from build123d import *

# Parameters (mm, degrees)
SKETCH1_W                          = 20
SKETCH1_H                          = 25
BOSS_EXTRUDE1_DEPTH                = 5
BOSS_EXTRUDE3_DEPTH                = 100
CUT_EXTRUDE2_DEPTH                 = 110.772492001
FILLET1_R                          = 3
SHELL1_START                       = 2.5
SHELL1_DEPTH                       = 13.421878312
SHELL1_START_2                     = 15.921878312
SHELL1_2_DEPTH                     = 86.578121688
SHELL1_START_3                     = 21.404196581
SHELL1_3_DEPTH                     = 2.5
M2_5X0_45_TAPPED_HOLE2_D           = 2.05
M2_5X0_45_TAPPED_HOLE2_CSINK_D     = 2.55
M2_5X0_45_TAPPED_HOLE2_CSINK_ANGLE = 90


with BuildPart() as part:
    # Sketch1 → Boss-Extrude1 (new body)
    with BuildSketch(Plane.XY):
        with Locations((10, 12.5)):
            Rectangle(SKETCH1_W, SKETCH1_H)
    extrude(amount=BOSS_EXTRUDE1_DEPTH)

    # Sketch2 → Boss-Extrude3 (add)
    with BuildSketch(Plane.XY.offset(5)):
        Polygon((0, 0), (0, 3.587380473), (9.227415524, 23.375636922), (10.227415524, 23.375636922), (20, 2.418261881), (20, 0), align=None)
    extrude(amount=BOSS_EXTRUDE3_DEPTH)

    # Sketch3 → Cut-Extrude2 (cut, through all)
    with BuildSketch(Plane(origin=(20, 0, 0), x_dir=(0, 0, -1), z_dir=(1, 0, 0))):
        Polygon((-105, 2.418261881), (-5, 23.375636922), (-105, 23.375636922), align=None)
    extrude(amount=-CUT_EXTRUDE2_DEPTH, mode=Mode.SUBTRACT)

    # Fillet1
    fillet1_edges = [part.edges().sort_by_distance(p)[0] for p in [
        (0, 25, 2.5),
        (20, 25, 2.5),
    ]]
    fillet(fillet1_edges, radius=FILLET1_R)

    # Shell1: read off the stored shape, not the designer's step
    # Shell1 outline → Shell1 (cut)
    with BuildSketch(Plane.XY.offset(SHELL1_START)):
        Polygon((2.5, 3.033143816), (2.5, 0), (17.5, 0), (17.5, 1.864025225), (9.727415524, 18.532386424), align=None)
    extrude(amount=SHELL1_DEPTH, mode=Mode.SUBTRACT)

    # Shell1 2 outline → Shell1 2 (cut)
    with BuildSketch(Plane.XY.offset(SHELL1_START_2)):
        Polygon((2.5, 3.033143816), (2.5, 0), (17.5, 0), (17.5, 1.864025225), (9.727415524, 18.532386424), align=None)
    extrude(amount=SHELL1_2_DEPTH, mode=Mode.SUBTRACT)

    # Shell1 3 outline → Shell1 3 (add)
    with BuildSketch(Plane(origin=(0, 0, 0), x_dir=(1, 0, 0), z_dir=(0, 0.9787373237991824, 0.2051176516110071)).offset(SHELL1_START_3)):
        Polygon((17.5, -93.044458657), (9.727415524, -11.782016987), (2.5, -87.344712281), (2.5, -100.241013679), (17.5, -100.241013679), align=None)
    extrude(amount=SHELL1_3_DEPTH)

    # M2.5x0.45 Tapped Hole2 (through all)
    with Locations(Plane.XY.offset(5)):
        with Locations((16, 18.307180682), (4, 18.307180682)):
            CounterSinkHole(M2_5X0_45_TAPPED_HOLE2_D / 2, M2_5X0_45_TAPPED_HOLE2_CSINK_D / 2, counter_sink_angle=M2_5X0_45_TAPPED_HOLE2_CSINK_ANGLE)


solid = part.part
Input: part model. Units: mm. Frame: model coordinates. A direction names the side the tool comes from. Coordinates: 2 decimals unless noted, no trailing zeros. Loops run counter-clockwise (first coordinate to the right, second up) from the corner with the lowest first, then second, coordinate; pieces in that order, holes last.
Q1. Draft query along Y for faces 1 (the face through (14.53, 8.23, 38)), 2 (the face through (4.2, 17.3, 2.3)), 3 (the face through (17.217, 8.386, 32.078)), 4 (the face through (0, 3, 44)). Return one class per face: +Y half, -Y half, draft (parallel to the pull), parting line (faces both ways), or undercut.
Q2. Contact query for flat-ended pins moving along their axis: pin 1 (1 mm diameter, centred on y = 7, z = 36, fed in from +X); pin 2 (10 mm diameter, centred on x = 12.5, z = 68.5, fed in from +Y); pin 3 (3 mm diameter, centred on y = 8.5, z = 22, fed in from +X). Output: stop coordinate, or through.
Q3. Material intervals for line 1 (Y direction, x = 4, z = 2.4); line 2 (X direction, y = 2.5, z = 80); line 3 (X direction, y = 5.5, z = 70.5), sorted ascending.
Q4. Cut plane B-B (y = 4.5). Output: boundary loops of the cut face in (x, z).
Q5. Cut plane C-C (z = 22). Output: boundary loops of the cut face in (x, y), then the cut area to 3 significant figures.
Q6. Cut plane D-D (x = 4). Output: boundary loops of the cut face in (y, z).
Q7. Cut plane A-A (x = 16). Output: boundary loops of the cut face in (y, z).
Q8. Set-up query: faces 5 (the face through (0.86, 24.1, 2.54)), 6 (the face through (9.895, 7.571, 68.225)), 7 (the face through (7.6, 21.4, 5)). Return all of +Z, -Z, +X, -X, +Y, -Y with unobstructed straight access to the full face (end or side cutting, diameter ignored); none if empty.
Working result:
1. face 1: -Y half
1. face 2: undercut
1. face 3: +Y half
1. face 4: draft
2. pin 1: stops at x = 18.1
2. pin 2: stops at y = 11.12
2. pin 3: stops at x = 17.86
3. line 1: y = 0 to 17.28, 19.33 to 25
3. line 2: x = 0 to 2.5, 17.2 to 19.96
3. line 3: x = 0.89 to 3.65, 15.8 to 18.56
4. outline: (0, 0) - (20, 0) - (20, 5) - (19.03, 5) - (19.03, 95.07) - (0.43, 95.07) - (0.43, 5) - (0, 5) - close; hole (3.18, 2.5) - (16.27, 2.5) - (16.27, 82.88) - (3.18, 82.88) - close
5. outline: (0, 0) - (2.5, 0) - (2.5, 3.03) - (9.13, 17.26) - (10.32, 17.26) - (17.5, 1.86) - (17.5, 0) - (20, 0) - (20, 2.42) - (11.89, 19.81) - (7.57, 19.81) - (0, 3.59) - close
5. area: 108 mm2
6. outline: (0, 0) - (17.28, 0) - (17.28, 4.75) - (17.03, 5) - (12.17, 5) - (12.17, 58.49) - (2.42, 105) - (0, 105) - (0, 102.5) - (0.39, 102.5) - (6.25, 74.53) - (6.25, 2.5) - (0, 2.5) - close; (19.33, 0) - (25, 0) - (25, 5) - (19.58, 5) - (19.33, 4.75) - close
7. outline: (0, 0) - (17.28, 0) - (17.28, 4.75) - (17.03, 5) - (11, 5) - (11, 64.07) - (2.42, 105) - (0, 105) - (0, 102.5) - (0.39, 102.5) - (5.08, 80.11) - (5.08, 2.5) - (0, 2.5) - close; (19.33, 0) - (25, 0) - (25, 5) - (19.58, 5) - (19.33, 4.75) - close
8. face 5: +Z, -Z, -X, +Y
8. face 6: -Y
8. face 7: +Z, +Y
